Geometry check sheet. Reference: the model listing, model coordinates, mm. Face numbers are marked on the shaded views. Coordinates: 2 decimals unless noted, no trailing zeros. Write each loop counter-clockwise with the first axis right and the second up, starting at its lowest first coordinate (ties: lowest second). Pieces come first, ordered by that corner, then holes.
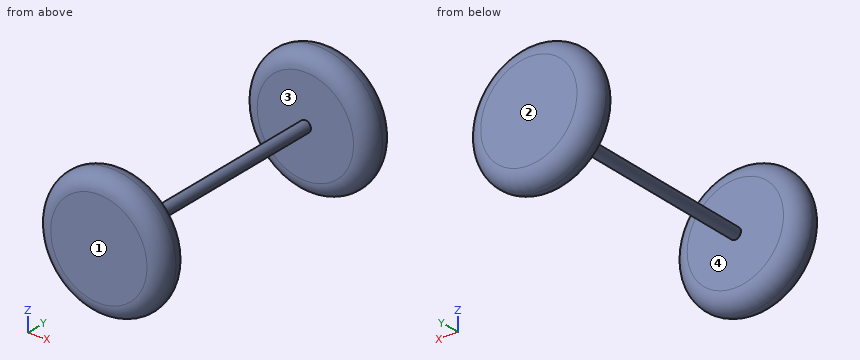
from build123d import *

# Parameters (mm, degrees)
F0_R     = 50.8
F1_DEPTH = 25.4
F2_R     = 12.7
F3_R     = 12.69999
F4_R     = 4.445
F5_DEPTH = 177.8
F6_R     = 50.8
F7_DEPTH = 25.4
F8_R     = 12.7
F9_R     = 12.69999


# Not quite as in the source:
# - a fillet or chamfer is up to 0.001 mm smaller than in the source, because OpenCascade refuses the exact size


with BuildPart() as f1:
    # F0 (on Front) → F1 (new body)
    with BuildSketch(Plane.XZ):
        Circle(F0_R)
    extrude(amount=F1_DEPTH)

    # F2
    f2_edges = [f1.edges().sort_by_distance(p)[0] for p in [
        (-50.8, -25.4, 0),
    ]]
    fillet(f2_edges, radius=F2_R)

    # F3 (radius 12.7 in the source; OpenCascade refuses exactly that, so slightly less here)
    f3_edges = [f1.edges().sort_by_distance(p)[0] for p in [
        (50.8, -6.35, 0),
        (-50.8, -12.7, 0),
        (-50.8, 0, 0),
    ]]
    fillet(f3_edges, radius=F3_R)

    # F4 (on face) → F5 (join)
    with BuildSketch(Plane(origin=(0, 0, 0), x_dir=(-1, 0, 0), z_dir=(0, 1, 0))):
        Circle(F4_R)
    extrude(amount=F5_DEPTH)

    # F6 (on face) → F7 (join)
    with BuildSketch(Plane(origin=(0, 177.8, 0), x_dir=(-1, 0, 0), z_dir=(0, 1, 0))):
        Circle(F6_R)
    extrude(amount=F7_DEPTH)

    # F8
    f8_edges = [f1.edges().sort_by_distance(p)[0] for p in [
        (50.8, 177.8, 0),
    ]]
    fillet(f8_edges, radius=F8_R)

    # F9 (radius 12.7 in the source; OpenCascade refuses exactly that, so slightly less here)
    f9_edges = [f1.edges().sort_by_distance(p)[0] for p in [
        (50.8, 203.2, 0),
    ]]
    fillet(f9_edges, radius=F9_R)


solid = f1.part
1. Sectioned sample at C-C, the plane y = 30.5. Record the boundary of the cut face in (x, z) (3 decimals), and give its area (3 significant figures).
Computed values:
outline: circle Ø8.89 at (0, 0)
area: 62.1 mm2
2. Gauge pin test, flat ends, axial feed: pin 1 Ø8 at (y, z) = (105, -1) entering from +X (3 decimals); pin 2 Ø4 at (x, z) = (-38.5, -29) entering from -Y. Record the tip position at first contact, or that the pin passes through.
Computed values:
pin 1: stops at x = 4.445
pin 2: stops at y = -22.48
3. Thickness scan on line 1 along Y through (x, z) = (-11, 12); line 2 along Y through (x, z) = (27, 28.5); line 3 along Z through (x, y) = (0, 109) (3 decimals). Record the ranges inside material, lowest first.
Computed values:
line 1: y = -25.4 to 0, 177.8 to 203.2
line 2: y = -25.35 to -0.05, 177.85 to 203.15
line 3: z = -4.445 to 4.445
4. Draft check along Y on the marked faces 1, 2, 3 and 4. Enter one of: released by +Y, released by -Y, zero draft, split by the parting line, or undercut.
Computed values:
face 1: released by -Y
face 2: released by +Y
face 3: undercut
face 4: undercut
5. Sectioned sample at D-D, the plane y = 188. Record the boundary of the cut face in (x, z).
Computed values:
outline: circle Ø101.1 at (0, 0)
